Autodesk Inventor part; units mm, degrees
ref_plane "YZ Plane" through (0, 0, 0) normal (1, 0, 0) x (0, 1, 0)
ref_plane "XZ Plane" through (0, 0, 0) normal (0, 1, 0) x (-1, 0, 0)
ref_plane "XY Plane" through (0, 0, 0) normal (0, 0, 1) x (1, 0, 0)
sketch "Sketch1" plane through (0, 0, 0) normal (0, 0, 1) x (1, 0, 0)
  circle A0 centre (0, 0) radius 50.8
  circle A1 centre (0, 0) radius 6.35
  line L0 (6.35, -3.6662) -> (0, -7.3323)
  line L1 (0, -7.3323) -> (-6.35, -3.6662)
  line L2 (-6.35, -3.6662) -> (-6.35, 3.6662)
  line L3 (-6.35, 3.6662) -> (0, 7.3323)
  line L4 (0, 7.3323) -> (6.35, 3.6662)
  line L5 (6.35, 3.6662) -> (6.35, -3.6662)
  point P0 (6.35, 0)
  dimension "d4" = 12.7
  dimension "d0" = 101.6
extrude "Extrusion1" add sketch "Sketch1" along normal blind 482.6
properties part number "4-bar intake roller"
Could you check a few things on this model? Use its own coordinates, in mm. Coordinates: 2 decimals unless noted, no trailing zeros. Order: outer loops, then holes, each group sorted by start corner. A loop starts at its lowest first (then second) coordinate and runs counter-clockwise, first axis right, second up.
Q1. Suppose I cut it at B-B on y = 20.5. Please give me the cut outline in (x, z).
Q2. Suppose I cut it at C-C on x = 16.5. Please give me the cut outline in (y, z).
Q3. Will these pins go through, and if not, where does the flat tip stop? pin 1 (10 mm diameter, centred on y = 26, z = 121, fed in from +X); pin 2 (12 mm diameter, centred on y = -18.5, z = 327.5, fed in from +X); pin 3 (12 mm diameter, centred on y = 11, z = 232.5, fed in from -X).
Q4. Please list where these lines run through material, in increasing order: L1, parallel to Y at x = -2, z = 447.5; L2, parallel to Y at x = -29, z = 186; L3, parallel to Y at x = 23, z = 314.
Q5. Suppose I cut it at A-A on z = 251.5. Please give me the cut outline in (x, y).
Answer:
1. outline: (-46.48, 0) - (46.48, 0) - (46.48, 482.6) - (-46.48, 482.6) - close
2. outline: (-48.05, 0) - (48.05, 0) - (48.05, 482.6) - (-48.05, 482.6) - close
3. pin 1: stops at x = 46.26
3. pin 2: stops at x = 49.24
3. pin 3: stops at x = -50.55
4. L1: y = -50.76 to -6.18, 6.18 to 50.76
4. L2: y = -41.71 to 41.71
4. L3: y = -45.3 to 45.3
5. outline: circle Ø101.6 at (0, 0); hole (-6.35, -3.67) - (0, -7.33) - (6.35, -3.67) - (6.35, 3.67) - (0, 7.33) - (-6.35, 3.67) - close
